Answer from the drawing. Dimensions are ordinates in mm from the lowest x, y and z of the part. A direction names the side the tool comes from. Round coordinates to 2 decimals unless told otherwise and drop trailing zeros. Write each loop counter-clockwise with the first axis right and the second up, starting at its lowest first coordinate (ties: lowest second). Pieces come first, ordered by that corner, then holes. Notation, with made-up numbers: (82.5, 78) - (133.5, 78) arc R15 cw to (133.5, 84) - close; hole circle Ø8 at (84.25, -29.75). An arc over 180 degrees is marked (long way). Answer in a Markdown table with one row per item.
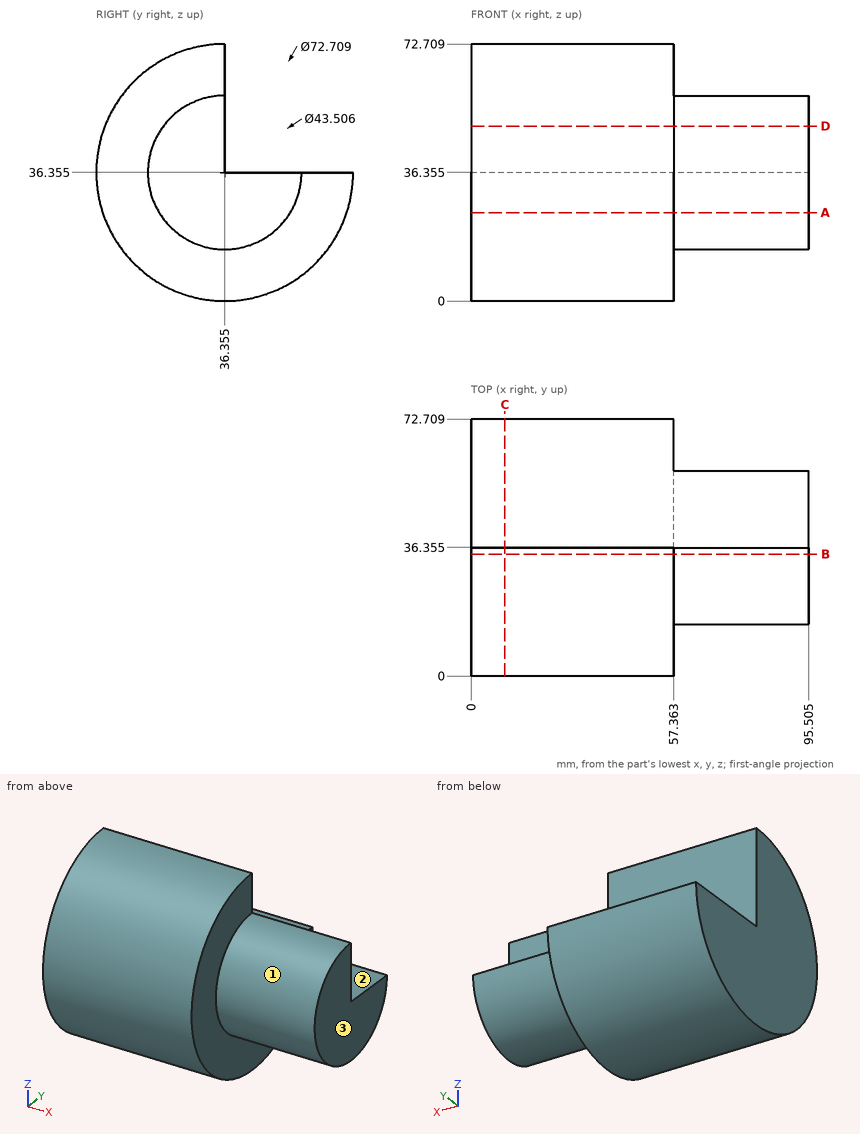
(1) Section B-B (y = 34.5) is taken. Give the vertices of the cut face in (x, z) (1 decimal), and give its area (3 significant figures).
Checked values:
| item | result |
|---|---|
| outline | (0, 0) - (57.4, 0) - (57.4, 14.7) - (95.5, 14.7) - (95.5, 58) - (57.4, 58) - (57.4, 72.7) - (0, 72.7) - close |
| area | 5,820 mm2 |
(2) Section D-D (z = 49.5) is taken. Give the vertices of the cut face in (x, y) (1 decimal).
Checked values:
| item | result |
|---|---|
| outline | (0, 2.5) - (57.4, 2.5) - (57.4, 19) - (95.5, 19) - (95.5, 36.4) - (0, 36.4) - close |
(3) Find the intervals of material crossed by line 1 (X direction, y = 37.5, z = 9); line 2 (Z direction, x = 60, y = 54) (1 decimal); line 3 (Z direction, x = 55, y = 9.5), in increasing order.
Checked values:
| item | result |
|---|---|
| line 1 | x = 0 to 57.36 |
| line 2 | z = 23.6 to 36.4 |
| line 3 | z = 11.85 to 60.86 |
(4) Flat-ended cylindrical pins translate along their axes: pin 1 (1 mm diameter, centred on y = 55.5, z = 19, fed in from +X); pin 2 (6 mm diameter, centred on x = 57, z = 16, fed in from +Y); pin 3 (5 mm diameter, centred on x = 16.5, y = 8, fed in from -Z). Find the tip coordinate at first contact, or state that the pin passes through.
Checked values:
| item | result |
|---|---|
| pin 1 | stops at x = 57.36 |
| pin 2 | stops at y = 68.3 |
| pin 3 | stops at z = 10.8 |
(5) Section A-A (z = 25) is taken. Give the vertices of the cut face in (x, y) (1 decimal).
Checked values:
| item | result |
|---|---|
| outline | (0, 1.8) - (57.4, 1.8) - (57.4, 17.8) - (95.5, 17.8) - (95.5, 54.9) - (57.4, 54.9) - (57.4, 70.9) - (0, 70.9) - close |
(6) For the marked faces 1, 2 and 3, determine the directions among +Z, -Z, +X, -X, +Y, -Y from which every point of the face is accessible in a straight line to the end or side of a thin tool.
Checked values:
| item | result |
|---|---|
| face 1 | +X |
| face 2 | +Z, +X, -X, +Y |
| face 3 | +Z, -Z, +X, +Y, -Y |
(7) Section C-C (x = 9.5) is taken. Give the vertices of the cut face in (y, z) (1 decimal), and give its area (3 significant figures).
Checked values:
| item | result |
|---|---|
| outline | (36.4, 36.4) - (36.4, 72.7) arc R36.4 ccw (long way) to (72.7, 36.4) - close |
| area | 3,110 mm2 |
